Design review of the part built by this model. Coordinates are the model's own, in mm. Give positions to 0.01 mm unless a question says otherwise; leave off trailing zeros. Loops run counter-clockwise (first coordinate to the right, second up) from the corner with the lowest first, then second, coordinate; pieces in that order, holes last. Notation, with made-up numbers: (-13.75, -31) -> (19.25, -31) arc R27 cw to (19.25, -10) -> close; hole circle Ø2 at (85, -11). An arc over 180 degrees is marked (long way). Answer in a Markdown table with one row per item. Add a question column.
(1) For line 1 (Y direction, x = 74, z = 12); line 2 (Y direction, x = 65.5, z = 16.75); line 3 (X direction, y = 125, z = 1.25), list the stretches that pass through material, from the lowest coordinate up.
(2) Draft analysis for pull direction X (two halves, no side actions). For faces 1 (the cylindrical face through (-199.69, -3.35, 21.58)), 2 (the cylindrical face through (154.305, 185.442, 12.522)), 3 (the cylindrical face through (-185.561, -184.923, 12.522)), 4 (the cylindrical face through (-2.137, 215.453, 3.819)), state which applies: +X half, -X half, draft (parallel to the pull), parting line (faces both ways), or undercut.
(3) Consider section A-A on z = 7.5. Write out the cut boundary in (x, y).
(4) For pin 1 (10 mm diameter, centred on x = 18, z = 4.5, fed in from +Y); pin 2 (1 mm diameter, centred on y = 104, z = 3, fed in from +X); pin 3 (4 mm diameter, centred on x = 134.5, y = -73.5, fed in from -Z); pin 4 (6 mm diameter, centred on x = 139, z = 21, fed in from +Y), all flat-tipped, find the tip position at first contact; note any pin that passes through.
from build123d import *

# Parameters (mm, degrees)
F1_DEPTH = 25.4
F2_R     = 12.69999


# Not quite as in the source:
# - a fillet or chamfer is up to 0.001 mm smaller than in the source, because OpenCascade refuses the exact size


with BuildPart() as f1:
    # F0 (on Top) → F1 (new body)
    with BuildSketch(Plane.XY):
        with BuildLine():
            ThreePointArc((-219.075, -183.3721313551), (-185.1905403178, -185.2885689585), (-183.4590722629, -219.182983829))
            Line((-183.4590722629, -219.182983829), (183.4590722629, -219.182983829))
            ThreePointArc((183.4590722629, -219.182983829), (185.1905403178, -185.2885689585), (219.075, -183.3721313551))
            Line((219.075, -183.3721313551), (187.072348327, 182.4198510941))
            ThreePointArc((187.072348327, 182.4198510941), (153.9534082329, 185.8090843811), (152.6381313551, 219.075))
            Line((152.6381313551, 219.075), (-152.6381313551, 219.075))
            ThreePointArc((-152.6381313551, 219.075), (-153.9534082329, 185.8090843811), (-187.072348327, 182.4198510941))
            Line((-187.072348327, 182.4198510941), (-219.075, -183.3721313551))
        make_face()
    extrude(amount=F1_DEPTH)

    # F2 (radius 12.7 in the source; OpenCascade refuses exactly that, so slightly less here)
    f2_edges = [f1.edges().sort_by_distance(p)[0] for p in [
        (-203.073674, -0.47614, 25.4),
        (0, 219.075, 25.4),
        (0, -219.182984, 25.4),
        (203.073674, -0.47614, 25.4),
        (-203.073674, -0.47614, 0),
        (0, -219.182984, 0),
        (0, 219.075, 0),
        (203.073674, -0.47614, 0),
    ]]
    fillet(f2_edges, radius=F2_R)


solid = f1.part
Values follow:
| question | item | result |
|---|---|---|
| 1 | line 1 | -219.16 to 219.06 |
| 1 | line 2 | -218.52 to 218.41 |
| 1 | line 3 | -184.86 to 184.86 |
| 2 | face 1 | -X half |
| 2 | face 2 | undercut |
| 2 | face 3 | undercut |
| 2 | face 4 | draft |
| 3 | outline | (-217.88, -182.47) arc R25.4 cw to (-182.61, -218.07) -> (182.61, -218.07) arc R25.4 cw to (217.88, -182.47) -> (186.02, 181.72) arc R25.4 cw to (151.8, 217.96) -> (-151.8, 217.96) arc R25.4 cw to (-186.02, 181.72) -> close |
| 4 | pin 1 | y = 218.67 |
| 4 | pin 2 | x = 189.97 |
| 4 | pin 3 | z = 0 |
| 4 | pin 4 | y = 217.92 |
